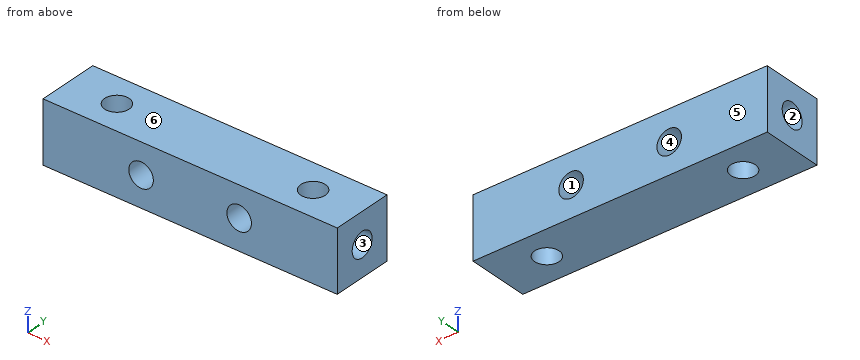
```python
from build123d import *

# Parameters (mm, degrees)
SKETCH_1_W          = 48
SKETCH_1_H          = 10
EXTRUDE_1_DEPTH     = 10
SKETCH_2_R          = 2
CUT_EXTRUDE_1_DEPTH = 10
SKETCH_3_R          = 2
CUT_EXTRUDE_2_DEPTH = 10
SKETCH_4_R          = 2
CUT_EXTRUDE_3_DEPTH = 8


with BuildPart() as part:
    # 草图1 → 凸台-拉伸1 (new body)
    with BuildSketch(Plane(origin=(0, 0, 0), x_dir=(1, 0, 0), z_dir=(0, 1, 0))):
        Rectangle(SKETCH_1_W, SKETCH_1_H)
    extrude(amount=EXTRUDE_1_DEPTH)

    # 草图2 → 切除-拉伸1 (cut)
    with BuildSketch(Plane.XY.offset(5)):
        with Locations((-16, 5)):
            Circle(SKETCH_2_R)
        with Locations((16, 5)):
            Circle(SKETCH_2_R)
    extrude(amount=-CUT_EXTRUDE_1_DEPTH, mode=Mode.SUBTRACT)

    # 草图3 → 切除-拉伸2 (cut)
    with BuildSketch(Plane(origin=(0, 10, 0), x_dir=(1, 0, 0), z_dir=(0, 1, 0))):
        with Locations(Location((-8, 0, 0), (0, 0, 270))):
            Circle(SKETCH_3_R)
        with Locations(Location((8, 0, 0), (0, 0, 270))):
            Circle(SKETCH_3_R)
    extrude(amount=-CUT_EXTRUDE_2_DEPTH, mode=Mode.SUBTRACT)

    # 草图4 → 切除-拉伸3 (cut)
    with BuildSketch(Plane.ZY.offset(24)):
        with Locations((0, 5)):
            Circle(SKETCH_4_R)
    cut_extrude_3 = extrude(amount=-CUT_EXTRUDE_3_DEPTH, mode=Mode.SUBTRACT)

    # 镜向1: 切除-拉伸3 across plane
    add(cut_extrude_3.mirror(Plane(origin=(0, 0, 0), x_dir=(0, 0, 1), z_dir=(1, 0, 0))), mode=Mode.SUBTRACT)


solid = part.part
```
Geometry: final body of the model. Coordinates: model frame, mm. Face numbers are marked on the shaded views. A direction names the side the tool comes from. Round coordinates to 2 decimals unless told otherwise and drop trailing zeros. Loops run counter-clockwise (first coordinate to the right, second up) from the corner with the lowest first, then second, coordinate; pieces in that order, holes last.
Item 1: Section A-A, the plane y = 5. Output: boundary loops of the cut face in (x, z), plus the area to 3 significant figures.
Checked values:
outline: (-24, -5) - (-18, -5) - (-18, -2) - (-24, -2) - close; (-24, 2) - (-18, 2) - (-18, 5) - (-24, 5) - close; (-14, -5) - (14, -5) - (14, 5) - (-14, 5) - close; (18, -5) - (24, -5) - (24, -2) - (18, -2) - close; (18, 2) - (24, 2) - (24, 5) - (18, 5) - close; hole circle Ø4 at (-8, 0); hole circle Ø4 at (8, 0)
area: 327 mm2
Item 2: Section C-C, the plane z = 0. Output: boundary loops of the cut face in (x, y), plus the area to 3 significant figures.
Checked values:
outline: (-24, 0) - (-10, 0) - (-10, 10) - (-24, 10) - (-24, 7) - (-16, 7) arc R2 cw to (-16, 3) - (-24, 3) - close; (-6, 0) - (6, 0) - (6, 10) - (-6, 10) - close; (10, 0) - (24, 0) - (24, 3) - (16, 3) arc R2 cw to (16, 7) - (24, 7) - (24, 10) - (10, 10) - close
area: 323 mm2
Item 3: Section D-D, the plane z = 3. Output: boundary loops of the cut face in (x, y), plus the area to 3 significant figures.
Checked values:
outline: (-24, 0) - (24, 0) - (24, 10) - (-24, 10) - close; hole circle Ø4 at (-16, 5); hole circle Ø4 at (16, 5)
area: 455 mm2
Item 4: Contact query for flat-ended pins moving along their axis: P1, Ø2.5, axis at x = 8, z = 0, coming from the -Y side; P2, Ø2.5, axis at y = 5, z = 0, coming from the -X side. Output: stop coordinate, or through.
Checked values:
P1: passes through
P2: stops at x = -14.44
Item 5: Reachability of the marked faces 1, 2 and 3 from +Z, -Z, +X, -X, +Y, -Y: full face, straight path, thin tool, end or side. Return the list, or none.
Checked values:
face 1: +Y, -Y
face 2: -X
face 3: +X
Item 6: Section B-B, the plane x = -8. Output: boundary loops of the cut face in (y, z), plus the area to 3 significant figures.
Checked values:
outline: (0, -5) - (10, -5) - (10, -2) - (0, -2) - close; (0, 2) - (10, 2) - (10, 5) - (0, 5) - close
area: 60.0 mm2
Item 7: Mould query, pull axis Z, two halves, no side actions, for the marked faces 4, 5 and 6. Classes: released by +Z, released by -Z, zero draft, split by the parting line, or undercut.
Checked values:
face 4: undercut
face 5: zero draft
face 6: released by +Z
Item 8: Line query: L1, parallel to X at y = 7.5, z = 0; L2, parallel to Z at x = -20, y = 5; L3, parallel to X at y = 4.5, z = -0.5. Output: solid intervals per line, ascending.
Checked values:
L1: x = -24 to -10, -6 to 6, 10 to 24
L2: z = -5 to -2, 2 to 5
L3: x = -14.06 to -9.94, -6.06 to 6.06, 9.94 to 14.06
